Autodesk Inventor part; units mm, degrees
ref_plane "YZ Plane" through (0, 0, 0) normal (1, 0, 0) x (0, 1, 0)
ref_plane "XZ Plane" through (0, 0, 0) normal (0, 1, 0) x (-1, 0, 0)
ref_plane "XY Plane" through (0, 0, 0) normal (0, 0, 1) x (1, 0, 0)
sketch "Sketch1" plane through (0, 0, 0) normal (0, 0, 1) x (1, 0, 0)
  line L0 (-51.9238, 7.67) -> (40.5487, 7.67)
  line L1 (50.9762, -5.53) -> (50.9762, -7.53)
  line L2 (50.9762, -7.53) -> (-51.9238, -7.53)
  line L3 (-51.9238, -7.53) -> (-51.9238, 7.67)
  line L4 (-51.9238, 7.67) -> (50.9762, -7.53) construction
  line L5 (50.8142, 7.3691) -> (-51.9238, -7.53) construction
  line L6 (40.55, -5.53) -> (50.9762, -5.53)
  line L7 (40.5487, 5.67) -> (-49.9238, 5.67)
  line L8 (-49.9238, 5.67) -> (-49.9238, 3.42)
  line L9 (-49.9238, 3.42) -> (38.3707, 3.42)
  line L10 (40.5487, 7.67) -> (40.5487, 5.8804)
  line L11 (40.55, -5.53) -> (-49.9238, -5.53)
  line L12 (-49.9238, -5.53) -> (-49.9238, -3.28)
  line L13 (-49.9238, -3.28) -> (38.3707, -3.28)
  line L14 (40.5487, 5.8804) -> (40.5487, 5.67)
  line L15 (38.3707, 2.82) -> (-49.9238, 2.82)
  line L16 (-49.9238, 2.82) -> (-49.9238, 0.57)
  line L17 (-49.9238, 0.57) -> (38.3707, 0.57)
  line L18 (38.3707, 3.42) -> (38.3707, 2.82)
  line L19 (38.3707, -0.03) -> (-49.9238, -0.03)
  line L20 (-49.9238, -0.03) -> (-49.9238, -2.28)
  line L21 (-49.9238, -2.28) -> (38.3707, -2.28)
  line L22 (38.3707, 0.57) -> (38.3707, -0.03)
  line L23 (38.3707, -2.28) -> (38.3707, -3.28)
  point P0 (0, 0)
  dimension "d0" = 102.9
  dimension "d1" = 14.9
  dimension "d3" = 2
  dimension "d4" = 2
  dimension "d5" = 2.25
  dimension "d6" = 2
  dimension "d7" = 2
  dimension "d8" = 2.25
  dimension "d10" = 0.6
  dimension "d11" = 2.25
  dimension "d12" = 2
  dimension "d13" = 0.6
  dimension "d14" = 2.25
  dimension "d15" = 1
  dimension "d16" = 2
extrude "Extrusion1" add sketch "Sketch1" along normal blind 54.5
sketch "Sketch2" plane through (0, 0, 54.5) normal (0, 0, 1) x (1, 0, 0)
  line L0 (-51.9238, 7.67) -> (40.5487, 7.67)
  line L1 (50.9762, -7.53) -> (-51.9238, -7.53)
  line L2 (40.5487, 7.67) -> (-51.9238, 7.67)
  line L3 (-51.9238, 7.67) -> (-51.9238, -7.53)
  line L4 (-51.9238, -7.53) -> (40.5487, -7.53)
  line L5 (40.5487, -7.53) -> (40.5487, 7.67)
  point P0 (0, 0)
extrude "Extrusion2" add sketch "Sketch2" along normal blind 2
sketch "Sketch3" plane through (0, 0, 0) normal (0, 0, -1) x (-1, 0, 0)
  line L0 (-40.5487, 7.67) -> (-40.5487, 5.67)
  line L1 (51.9238, -7.53) -> (51.9238, 7.67)
  line L2 (-40.5487, 7.67) -> (51.9238, 7.67)
  line L3 (51.9238, 7.67) -> (51.9238, -7.53)
  line L4 (51.9238, -7.53) -> (-40.5487, -7.53)
  line L5 (-40.5487, -7.53) -> (-40.5487, 7.67)
  point P0 (0, 0)
extrude "Extrusion3" add sketch "Sketch3" along normal blind 2
sketch "Sketch4" plane through (40.5487, -7.53, 0) normal (0, -1, 0) x (1, 0, 0)
  line L0 (8.4275, 31.25) -> (2.4275, 31.25)
  line L1 (2.4275, 31.25) -> (2.4275, 23.25)
  line L2 (2.4275, 23.25) -> (8.4275, 23.25)
  line L3 (8.4275, 23.25) -> (8.4275, 31.25)
  line L4 (10.4275, 0) -> (10.4275, 54.5)
  line L5 (10.4275, 0) -> (0, 0)
  point P0 (-40.5487, 0)
  dimension "d23" = 2
  dimension "d24" = 8
  dimension "d25" = 6
  dimension "d26" = 23.25
extrude "Extrusion4" cut sketch "Sketch4" against normal blind 2
chamfer "Chamfer1" distance 2 angle 45 10 edges at (-5.6875, 7.67, -2) (-5.6875, -7.53, -2) (-51.9238, 0.07, -2) (-51.9238, 7.67, 27.25) (-5.6875, 7.67, 56.5) (-51.9238, -7.53, 27.25) (-5.6875, -7.53, 56.5) (-51.9238, 0.07, 56.5) (40.5487, 0.07, -2) (40.5487, 0.07, 56.5)
properties part number "CardBox_4slots_template"
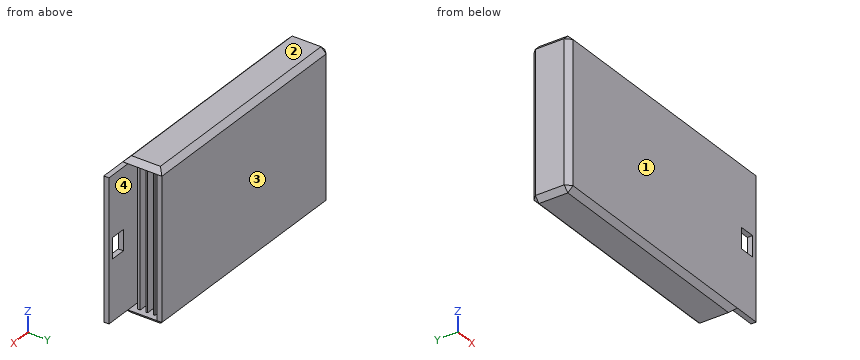
Can you work these out from the model? Positions are in its coordinate system, mm. Face numbers are marked on the shaded views. Round coordinates to 2 decimals unless told otherwise and drop trailing zeros. Loops run counter-clockwise (first coordinate to the right, second up) from the corner with the lowest first, then second, coordinate; pieces in that order, holes last. Notation, with made-up numbers: (7, 6.25) -> (62, 6.25) arc R29 ccw to (62, 39.25) -> close; hole circle Ø10 at (4.5, 89). An arc over 180 degrees is marked (long way). One line per item, written item: value. Start each with the question number.
1. If we mould it in two halves opening along Y, with no side actions, what happens to the marked faces 1, 2, 3 and 4? For each: pulls with the +Y half, pulls with the -Y half, needs draft (parallel to the pull), parting line crosses it, or undercut.
2. If we section it at B-B, the plane z = 27: Write out the boundary of the cut face in (x, y), then the cut area to 3 significant figures.
3. For pin 1 (1 mm diameter, centred on x = 46.5, y = -6.5, fed in from +Z); pin 2 (0.7 mm diameter, centred on y = 0, z = 26, fed in from +X); pin 3 (1.1 mm diameter, centred on y = -1.5, z = 16.5, fed in from +X), each with a flat end and sliding along its axis, tell me the tip position at first contact or that it passes through.
4. If we section it at D-D, the plane z = 52: Write out the boundary of the cut face in (x, y).
5. If I drill on probe 1 along Y at (x, z) = (-25.5, 4); probe 2 along Z at (x, y) = (-36, 1.5); probe 3 along Z at (x, y) = (45, -6), over which ranges is the centre line in solid material (lowest first)?
6. If we section it at A-A, the plane x = 4: Write out the boundary of the cut face in (y, z).
Calculated:
1. face 1: pulls with the -Y half
1. face 2: needs draft
1. face 3: pulls with the +Y half
1. face 4: undercut
2. outline: (-51.92, -5.53) -> (-49.92, -7.53) -> (42.98, -7.53) -> (42.98, -5.53) -> (-49.92, -5.53) -> (-49.92, -3.28) -> (38.37, -3.28) -> (38.37, -2.28) -> (-49.92, -2.28) -> (-49.92, -0.03) -> (38.37, -0.03) -> (38.37, 0.57) -> (-49.92, 0.57) -> (-49.92, 2.82) -> (38.37, 2.82) -> (38.37, 3.42) -> (-49.92, 3.42) -> (-49.92, 5.67) -> (40.55, 5.67) -> (40.55, 7.67) -> (-49.92, 7.67) -> (-51.92, 5.67) -> close; (48.98, -7.53) -> (50.98, -7.53) -> (50.98, -5.53) -> (48.98, -5.53) -> close
2. area: 591 mm²
3. pin 1: stops at z = 54.5
3. pin 2: stops at x = 38.37
3. pin 3: stops at x = -49.92
4. outline: (-51.92, -5.53) -> (-49.92, -7.53) -> (50.98, -7.53) -> (50.98, -5.53) -> (-49.92, -5.53) -> (-49.92, -3.28) -> (38.37, -3.28) -> (38.37, -2.28) -> (-49.92, -2.28) -> (-49.92, -0.03) -> (38.37, -0.03) -> (38.37, 0.57) -> (-49.92, 0.57) -> (-49.92, 2.82) -> (38.37, 2.82) -> (38.37, 3.42) -> (-49.92, 3.42) -> (-49.92, 5.67) -> (40.55, 5.67) -> (40.55, 7.67) -> (-49.92, 7.67) -> (-51.92, 5.67) -> close
5. probe 1: y = -7.53 to -5.53, -3.28 to -2.28, -0.03 to 0.57, 2.82 to 3.42, 5.67 to 7.67
5. probe 2: z = -2 to 0, 54.5 to 56.5
5. probe 3: z = 0 to 23.25, 31.25 to 54.5
6. outline: (-7.53, 0) -> (-5.53, -2) -> (5.67, -2) -> (7.67, 0) -> (7.67, 54.5) -> (5.67, 56.5) -> (-5.53, 56.5) -> (-7.53, 54.5) -> close; hole (-5.53, 0) -> (-3.28, 0) -> (-3.28, 54.5) -> (-5.53, 54.5) -> close; hole (-2.28, 0) -> (-0.03, 0) -> (-0.03, 54.5) -> (-2.28, 54.5) -> close; hole (0.57, 0) -> (2.82, 0) -> (2.82, 54.5) -> (0.57, 54.5) -> close; hole (3.42, 0) -> (5.67, 0) -> (5.67, 54.5) -> (3.42, 54.5) -> close
